from build123d import *

# Parameters (mm, degrees)
F1_DEPTH = 5
F2_R     = 1.25
F3_DEPTH = 6
F5_R     = 1.25
F6_DEPTH = 7


with BuildPart() as f1:
    # F0 (on Top) → F1 (new body)
    with BuildSketch(Plane.XY):
        Polygon((1.379062, -2.379225), (2.75, 0.00469), (1.370938, 2.383915), (-1.379062, 2.379225), (-2.75, -0.00469), (-1.370938, -2.383915), align=None)
    extrude(amount=F1_DEPTH)

    # F2 (on Top) → F3 (join)
    with BuildSketch(Plane.XY):
        Circle(F2_R)
    extrude(amount=-F3_DEPTH)

    # F5 (on offset) → F6 (cut)
    with BuildSketch(Plane.XY.offset(4)):
        Circle(F5_R)
    extrude(amount=F6_DEPTH, mode=Mode.SUBTRACT)


solid = f1.part
Model file for the job. Use its own axes, mm. A direction names the side the tool comes from. Give positions to 0.01 mm unless a question says otherwise; leave off trailing zeros. Order: outer loops, then holes, each group sorted by start corner. A loop starts at its lowest first (then second) coordinate and runs counter-clockwise, first axis right, second up. Notation, with made-up numbers: (55.25, 30.25) - (110.25, 30.25) arc R30 ccw to (110.25, 52.25) - close; hole circle Ø8 at (-13, 33). An arc over 180 degrees is marked (long way). Return JSON: item names as keys, results as strings.
1) Cut at C-C, the plane y = 1.45. Give the cut face in (x, z), plus the area to 3 significant figures.
Geometry says:
{"outline": "(-1.91, 0) - (1.91, 0) - (1.91, 5) - (-1.91, 5) - close", "area": "19.1 mm²"}
2) Cut at D-D, the plane z = -1.75. Give the cut face in (x, y), plus the area to 3 significant figures.
Geometry says:
{"outline": "circle Ø2.5 at (0, 0)", "area": "4.91 mm²"}
3) Cut at A-A, the plane z = 3.5. Give the cut face in (x, y), plus the area to 3 significant figures.
Geometry says:
{"outline": "(-2.75, 0) - (-1.37, -2.38) - (1.38, -2.38) - (2.75, 0) - (1.37, 2.38) - (-1.38, 2.38) - close", "area": "19.6 mm²"}
4) Probe line 1 (Y direction, x = 0, z = 4.4); line 2 (Y direction, x = 1.15, z = 0.25); line 3 (Z direction, x = 2.3, y = 0.15). List the from-to ranges inside material, lowest first. Write a range as from..to.
Geometry says:
{"line 1": "-2.38..-1.25, 1.25..2.38", "line 2": "-2.38..2.38", "line 3": "0..5"}
5) Flat gauge pins, fed straight in: P1, Ø1.5, axis at y = -1.5, z = 1, coming from the -X side; P2, Ø1, axis at y = -1, z = 1, coming from the -X side. Where does each tip first touch, or does it go through?
Geometry says:
{"P1": "x = -2.32", "P2": "x = -2.46"}
6) Cut at B-B, the plane x = 0. Give the cut face in (y, z).
Geometry says:
{"outline": "(-2.38, 0) - (-1.25, 0) - (-1.25, -6) - (1.25, -6) - (1.25, 0) - (2.38, 0) - (2.38, 5) - (1.25, 5) - (1.25, 4) - (-1.25, 4) - (-1.25, 5) - (-2.38, 5) - close"}
7) Pull direction X, two halves, no side cores. Call faces 3 (the flat face through (1, 1, 0)), 4 (the flat face through (2.07, 1.18, 2.46)), 5 (the flat face through (0, 0, 4)), 6 (the cylindrical face through (-0.27, -1.22, -2.96)): pulls with the +X half, pulls with the -X half, needs draft (parallel to the pull), parting line crosses it, or undercut.
Geometry says:
{"face 3": "needs draft", "face 4": "pulls with the +X half", "face 5": "undercut", "face 6": "parting line crosses it"}
8) 3-axis set-ups, long thin cutter, end or side, ignore diameter. For faces 1 (the cylindrical face through (-0.27, -1.22, 4.49)), 2 (the flat face through (2.055, -1.204, 2.465)): which of +Z, -Z, +X, -X, +Y, -Y reach the whole face in a straight line?
Geometry says:
{"face 1": "+Z", "face 2": "+Z, -Z, +X, -Y"}
